Verification items for the finished model (mm, model axes). Give positions to 0.01 mm unless a question says otherwise; leave off trailing zeros. Order: outer loops, then holes, each group sorted by start corner. A loop starts at its lowest first (then second) coordinate and runs counter-clockwise, first axis right, second up.
(1) Scan lines: L1, parallel to Y at x = 18, z = -241.29; L2, parallel to X at y = -0.25, z = -236; L3, parallel to Y at x = 2.5, z = 0. Record each from-to range of solid material in increasing order.
(2) Sectioned sample at A-A on y = -6. Record the cut outline in (x, z).
(3) Gauge pin test, flat ends, axial feed: pin 1 (8 mm diameter, centred on x = 1, y = -12.5, fed in from +Z); pin 2 (14 mm diameter, centred on x = 1.5, z = -78, fed in from +Y); pin 3 (1.5 mm diameter, centred on y = -2, z = -177, fed in from +X); pin 4 (8 mm diameter, centred on y = -6, z = 0, fed in from +X). Record the tip position at first contact, or that the pin passes through.
(4) Sectioned sample at D-D on x = 18.25. Record the cut outline in (y, z), plus the area to 3 significant figures.
(5) Sectioned sample at B-B on z = 0. Record the cut outline in (x, y).
(6) Sectioned sample at C-C on z = -241.29. Record the cut outline in (x, y).
```python
from build123d import *

# Parameters (mm, degrees)
BOSS_EXTRUDE1_DEPTH = 12
CUT_EXTRUDE3_REACH  = 251.216
SKETCH2_R           = 5
CUT_EXTRUDE4_REACH  = 251.216
SKETCH3_R           = 3.5
SKETCH4_R           = 10
SKETCH4_R_2         = 5
BOSS_EXTRUDE2_DEPTH = 12


with BuildPart() as part:
    # Sketch1 → Boss-Extrude1 (new body)
    with BuildSketch(Plane(origin=(0, 0, 0), x_dir=(1, 0, 0), z_dir=(0, 1, 0))):
        Polygon((10.5, 227.29), (22.5, 227.29), (6, 14), (-6, 14), align=None)
        Polygon((22.5, 227.29), (22.5, 241.29), (22.5, 247.29), (16.5, 247.29), (10.5, 247.29), (10.5, 227.29), align=None)
        Polygon((6, -6), (6, 14), (-6, 14), (-6, 0), (-6, -6), (0, -6), align=None)
    extrude(amount=-BOSS_EXTRUDE1_DEPTH)

    # Sketch2 → Cut-Extrude3 (cut, up to next)
    with BuildSketch(Plane.ZY.offset(6), mode=Mode.PRIVATE) as cut_extrude3_sk1:
        with Locations((0, -6)):
            Circle(SKETCH2_R)
    cut_extrude3_tool1 = extrude(cut_extrude3_sk1.sketch, amount=-CUT_EXTRUDE3_REACH, mode=Mode.PRIVATE) & part.part
    add(cut_extrude3_tool1.solids().sort_by_distance((-6, -6, 0))[0], mode=Mode.SUBTRACT)

    # Sketch3 → Cut-Extrude4 (cut, up to next)
    with BuildSketch(Plane(origin=(22.5, 0, 0), x_dir=(0, 0, -1), z_dir=(1, 0, 0)), mode=Mode.PRIVATE) as cut_extrude4_sk1:
        with Locations((241.29, -6)):
            Circle(SKETCH3_R)
    cut_extrude4_tool1 = extrude(cut_extrude4_sk1.sketch, amount=-CUT_EXTRUDE4_REACH, mode=Mode.PRIVATE) & part.part
    add(cut_extrude4_tool1.solids().sort_by_distance((22.5, -6, -241.29))[0], mode=Mode.SUBTRACT)

    # Sketch4 → Boss-Extrude2 (add)
    with BuildSketch(Plane.ZY.offset(6)):
        with Locations((0, -6)):
            Circle(SKETCH4_R)
        with Locations((0, -6)):
            Circle(SKETCH4_R_2, mode=Mode.SUBTRACT)
    extrude(amount=-BOSS_EXTRUDE2_DEPTH)


solid = part.part
```
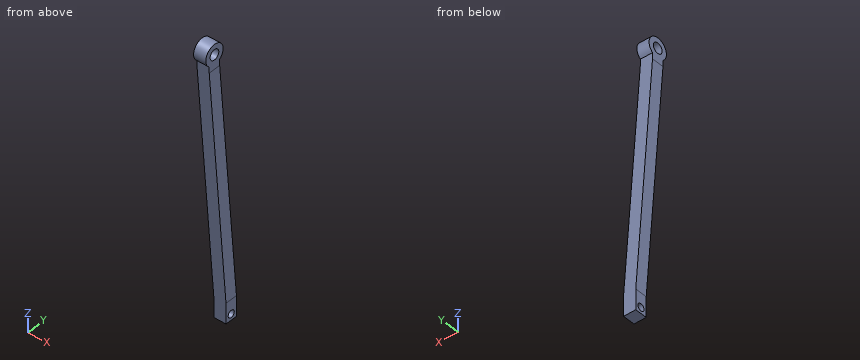
Ans:
1. L1: y = -12 to -9.5, -2.5 to 0
1. L2: x = 10.5 to 22.5
1. L3: y = -16 to -11, -1 to 4
2. outline: (-6, -14) - (10.5, -227.29) - (10.5, -237.79) - (22.5, -237.79) - (22.5, -227.29) - (6, -14) - (6, -5) - (-6, -5) - close; (-6, 5) - (6, 5) - (6, 10) - (-6, 10) - close; (10.5, -247.29) - (22.5, -247.29) - (22.5, -244.79) - (10.5, -244.79) - close
3. pin 1: stops at z = 9.68
3. pin 2: stops at y = 0
3. pin 3: stops at x = 18.67
3. pin 4: passes through
4. outline: (-12, -247.29) - (0, -247.29) - (0, -172.35) - (-12, -172.35) - close; hole circle Ø7 at (-6, -241.29)
4. area: 861 mm2
5. outline: (-6, -16) - (6, -16) - (6, -11) - (-6, -11) - close; (-6, -1) - (6, -1) - (6, 4) - (-6, 4) - close
6. outline: (10.5, -12) - (22.5, -12) - (22.5, -9.5) - (10.5, -9.5) - close; (10.5, -2.5) - (22.5, -2.5) - (22.5, 0) - (10.5, 0) - close
